Geometry: final body of the model. Coordinates: model frame, mm. A direction names the side the tool comes from. Give positions to 0.01 mm unless a question says otherwise; leave off trailing zeros. Order: outer loops, then holes, each group sorted by start corner. A loop starts at its lowest first (then second) coordinate and runs counter-clockwise, first axis right, second up. Notation, with made-up numbers: (-3.5, -2) -> (52.5, -2) arc R21 ccw to (52.5, 7) -> close; hole circle Ø5 at (0.25, -35). An arc over 180 degrees is marked (long way). One line per question, with ' | ' between items.
from build123d import *

# Parameters (mm, degrees)
F0_W      = 41
F0_H      = 98
F1_DEPTH  = 63
F3_DEPTH  = 9
F5_DEPTH  = 16
F7_DEPTH  = 98.001
F9_W      = 13
F9_H      = 51
F10_DEPTH = 63.001
F11_R     = 25.375
F12_DEPTH = 13
F13_R     = 11
F14_DEPTH = 5
F18_DEPTH = 41.001
F15_R     = 7.125
F19_DEPTH = 8
F22_DEPTH = 8
F23_W     = 14
F23_H     = 5
F24_DEPTH = 41.001
F25_R     = 4.5
F26_DEPTH = 32.001
F27_R     = 5.5
F28_DEPTH = 63.001


with BuildPart() as f1:
    # F0 (on Top) → F1 (new body)
    with BuildSketch(Plane.XY):
        Rectangle(F0_W, F0_H)
    extrude(amount=F1_DEPTH)

    # F2 (on face) → F3 (cut)
    with BuildSketch(Plane.YZ.offset(20.5)):
        with BuildLine():
            Line((27, 63), (27, 35))
            ThreePointArc((27, 35), (33.4436508139, 19.4436508139), (49, 13))
            Line((49, 13), (49, 63))
            Line((49, 63), (27, 63))
        make_face()
    extrude(amount=-F3_DEPTH, mode=Mode.SUBTRACT)

    # F4 (on face) → F5 (cut)
    with BuildSketch(Plane.XY.offset(63)):
        Polygon((11.5, 49), (-20.5, 49), (-20.5, 14), (20.5, 14), (20.5, 27), (11.5, 27), align=None)
    extrude(amount=-F5_DEPTH, mode=Mode.SUBTRACT)

    # F6 (on face) → F7 (cut, through all)
    with BuildSketch(Plane.XZ.offset(49)):
        Polygon((-20.5, 63), (-20.5, 49), (-12.4170962313, 63), align=None)
    extrude(amount=-F7_DEPTH, mode=Mode.SUBTRACT)

    # F9 (on offset) → F10 (cut, through all)
    with BuildSketch(Plane.XY.offset(63)):
        with Locations((-14, 23.5)):
            Rectangle(F9_W, F9_H)
    extrude(amount=-F10_DEPTH, mode=Mode.SUBTRACT)

    # F11 (on face) → F12 (cut)
    with BuildSketch(Plane.YZ.offset(20.5)):
        with Locations((-20, 30.8340992779)):
            Circle(F11_R)
    extrude(amount=-F12_DEPTH, mode=Mode.SUBTRACT)

    # F13 (on face) → F14 (join)
    with BuildSketch(Plane.YZ.offset(7.5)):
        with Locations((-20, 30.8340992779)):
            Circle(F13_R)
    extrude(amount=F14_DEPTH)

    # F17 (on offset) → F18 (cut, through all)
    with BuildSketch(Plane(origin=(-20.5, 0, 0), x_dir=(0, -1, 0), z_dir=(-1, 0, 0))):
        with BuildLine():
            Line((20, 63), (20, 35))
            ThreePointArc((20, 35), (68.2520480507, 7.4342434503), (67.4919333848, 63))
            Line((67.4919333848, 63), (20, 63))
        make_face()
    extrude(amount=-F18_DEPTH, mode=Mode.SUBTRACT)

    # F15 (on face) → F19 (join)
    with BuildSketch(Plane.YZ.offset(12.5)):
        with Locations((-20, 30.8340992779)):
            Circle(F15_R)
    extrude(amount=F19_DEPTH)

    # F21 (on offset) → F22 (join)
    with BuildSketch(Plane.YZ.offset(20.5)):
        with BuildLine():
            ThreePointArc((-36.1440872593, 11.2570956367), (-42.3689524888, 8.8269373419), (-49, 8))
            Line((-49, 8), (-49, 0))
            Line((-49, 0), (-33.1566682197, 0))
            Line((-33.1566682197, 0), (-33.1566682197, 9.1363411827))
            ThreePointArc((-33.1566682197, 9.1363411827), (-34.6887020452, 10.1427325461), (-36.1440872593, 11.2570956367))
        make_face()
    extrude(amount=-F22_DEPTH)

    # F23 (on face) → F24 (cut, through all)
    with BuildSketch(Plane.YZ.offset(20.5)):
        with Locations((10, 2.5)):
            Rectangle(F23_W, F23_H)
    extrude(amount=-F24_DEPTH, mode=Mode.SUBTRACT)

    # F25 (on face) → F26 (cut, through all)
    with BuildSketch(Plane.YZ.offset(11.5)):
        with Locations((38, 35)):
            Circle(F25_R)
    extrude(amount=-F26_DEPTH, mode=Mode.SUBTRACT)

    # F27 (on face) → F28 (cut, through all)
    with BuildSketch(Plane.XY.offset(63)):
        with Locations((-4.5, -11)):
            Circle(F27_R)
    extrude(amount=-F28_DEPTH, mode=Mode.SUBTRACT)


solid = f1.part
1) Section A-A on x = 5.5. Return loops of the section in (y, z), plus the area to 3 significant figures.
Check result:
outline: (-49, 0) -> (3, 0) -> (3, 5) -> (17, 5) -> (17, 0) -> (49, 0) -> (49, 47) -> (14, 47) -> (14, 63) -> (-20, 63) -> (-20, 35) arc R32 cw to (-49, 3.14) -> close; hole circle Ø9 at (38, 35) | area: 3,960 mm^2
2) Contact query for flat-ended pins moving along their axis: pin 1 Ø12 at (x, y) = (-14, 35) entering from +Z (1 decimal); pin 2 Ø4 at (y, z) = (-37.5, 6.5) entering from -X; pin 3 Ø17.5 at (x, z) = (0, 57.5) entering from +Y; pin 4 Ø6 at (x, y) = (-6, 18) entering from +Z. Output: stop coordinate, or through.
Check result:
pin 1: passes through | pin 2: stops at x = -20.5 | pin 3: stops at y = 14 | pin 4: stops at z = 47
3) Section D-D on z = 43. Return loops of the section in (x, y).
Check result:
outline: (-20.5, -20) -> (7.5, -20) -> (7.5, 2.27) -> (20.5, 2.27) -> (20.5, 27) -> (11.5, 27) -> (11.5, 49) -> (-7.5, 49) -> (-7.5, -2) -> (-20.5, -2) -> close; hole circle Ø11 at (-4.5, -11)
4) Set-up query: faces 1 (the flat face through (6, 14, 55)), 2 (the flat face through (7, 10, 5)), 3 (the flat face through (12.5, -24, 31)), 4 (the flat face through (7.5, -9.9, 25.6)). Return all of +Z, -Z, +X, -X, +Y, -Y with unobstructed straight access to the full face (end or side cutting, diameter ignored); none if empty.
Check result:
face 1: +Z, +X, -X, +Y | face 2: -Z, +X, -X | face 3: +Z, -X, -Y | face 4: +X
5) Pull-direction query (X, two-part tool) for faces 5 (the cylindrical face through (9.96, -9.19, 28.79)), 6 (the flat face through (-7.5, 23, 25)), 7 (the cylindrical face through (-5.69, -16.37, 31.94)); classes: +X half, -X half, draft (parallel to the pull), parting line (faces both ways), or undercut.
Check result:
face 5: draft | face 6: -X half | face 7: undercut
6) Material intervals for probe 1 along Z at (x, y) = (3, 38); probe 2 along X at (y, z) = (23, 13.5); probe 3 along Y at (x, z) = (-4.5, 56), sorted ascending. Write a range as from..to.
Check result:
probe 1: z = 0..30.5, 39.5..47 | probe 2: x = -7.5..20.5 | probe 3: y = -20..-16.5, -5.5..14
7) Section B-B on x = -4.5. Return loops of the section in (y, z), plus the area to 3 significant figures.
Check result:
outline: (-49, 0) -> (-16.5, 0) -> (-16.5, 63) -> (-20, 63) -> (-20, 35) arc R32 cw to (-49, 3.14) -> close; (-5.5, 0) -> (3, 0) -> (3, 5) -> (17, 5) -> (17, 0) -> (49, 0) -> (49, 47) -> (14, 47) -> (14, 63) -> (-5.5, 63) -> close; hole circle Ø9 at (38, 35) | area: 3,270 mm^2
8) Section C-C on y = 34.5. Return loops of the section in (x, z), plus the area to 3 significant figures.
Check result:
outline: (-7.5, 0) -> (20.5, 0) -> (20.5, 18.45) -> (11.5, 18.45) -> (11.5, 32.17) -> (-7.5, 32.17) -> close; (-7.5, 37.83) -> (11.5, 37.83) -> (11.5, 47) -> (-7.5, 47) -> close | area: 952 mm^2
